Build history of the part. All positions in model axes, mm. A direction names the side the tool comes from. Give positions to 0.01 mm unless a question says otherwise; leave off trailing zeros. Loops run counter-clockwise (first coordinate to the right, second up) from the corner with the lowest first, then second, coordinate; pieces in that order, holes last.
1) Band-saw the part on C-C on y = -3. List the corners of the cut face in (x, z), then the cut area to 3 significant figures.
2) 3-axis set-ups, long thin cutter, end or side, ignore diameter. For faces 1 (the flat face through (0, 0, 15)), 2 (the flat face through (15, 1, -2)), 3 (the flat face through (3.59, 11.248, -11.084)): which of +Z, -Z, +X, -X, +Y, -Y reach the whole face in a straight line?
3) Wall check: line 1 (X direction, y = -3.1, z = 22.45); line 2 (Z direction, x = 0, y = -4.2); line 3 (Z direction, x = 0, y = -3.5). Give the ranges that are in metal, low to high.
4) Band-saw the part on B-B on x = 0. State how many separate pieces and enclosed holes the cut face has, then the cut area to 3 significant figures.
5) Two-plate mould, pull along Y, no slides. Class faces 4 (the flat face through (0.21, 7.314, -6.137)), 5 (the flat face through (0, -2, 30)), 6 (the cylindrical face through (-0.145, 9.063, -8.439)): +Y half, -Y half, draft (parallel to the pull), parting line (faces both ways), or undercut.
6) Band-saw the part on A-A on z = 22.45. List the corners of the cut face in (x, y), then the cut area to 3 significant figures.
7) Flat gauge pins, fed straight in: P1, Ø5, axis at x = -7, z = -0.5, coming from the +Y side; P2, Ø1, axis at y = 3.5, z = -15.5, coming from the -X side; P3, Ø9, axis at x = 4.5, z = 16, coming from the +Y side; P4, Ø2, axis at x = -2, z = -17, coming from the -Y side. Where does each tip first touch, or does it go through?
```python
from build123d import *

# Parameters (mm, degrees)
SKETCH1_W                                           = 30
SKETCH1_H                                           = 5
BOSS_EXTRUDE1_DEPTH                                 = 30
BOSS_EXTRUDE3_DEPTH                                 = 30
CSK_FOR_M4_COUNTERSUNK_FLAT_HEAD_SCREW1_D           = 4.5
CSK_FOR_M4_COUNTERSUNK_FLAT_HEAD_SCREW1_CSINK_D     = 9.4
CSK_FOR_M4_COUNTERSUNK_FLAT_HEAD_SCREW1_CSINK_ANGLE = 90


with BuildPart() as part:
    # Sketch1 → Boss-Extrude1 (new body)
    with BuildSketch(Plane.XY):
        with Locations((0, -2.5)):
            Rectangle(SKETCH1_W, SKETCH1_H)
    extrude(amount=BOSS_EXTRUDE1_DEPTH)

    # Sketch3 → Boss-Extrude3 (add)
    with BuildSketch(Plane(origin=(15, 0, 0), x_dir=(0, 0, -1), z_dir=(1, 0, 0))):
        Polygon((0, 0), (16.069690242, 19.151111078), (26.069690242, 19.151111078), (5.804501844, -5), (0, -5), align=None)
    extrude(amount=-BOSS_EXTRUDE3_DEPTH)

    # Sketch6 → CBORE for M6 Hex Socket Head Cap Screw1 (revolve, cut)
    with BuildSketch(Plane(origin=(0, 7.075555539, -15.937096043), x_dir=(0, 0.766044443, -0.64278761), z_dir=(1, 0, 0))):
        Polygon((0, 0), (0, 42.951874637), (3.3, 42.951874637), (3.3, 6.4), (5.5, 6.4), (5.5, 0.025), (5.525, 0), align=None)
    revolve(axis=Axis((0, 2.993854217, -20.801478257), (0, 0.64278761, 0.766044443)), mode=Mode.SUBTRACT)

    # CSK for M4 Countersunk Flat Head Screw1 (through all)
    with Locations(Plane(origin=(0, 0, 0), x_dir=(1, 0, 0), z_dir=(0, 1, 0))):
        with Locations((0, -7.55), (0, -22.45)):
            CounterSinkHole(CSK_FOR_M4_COUNTERSUNK_FLAT_HEAD_SCREW1_D / 2, CSK_FOR_M4_COUNTERSUNK_FLAT_HEAD_SCREW1_CSINK_D / 2, counter_sink_angle=CSK_FOR_M4_COUNTERSUNK_FLAT_HEAD_SCREW1_CSINK_ANGLE)


solid = part.part
```
Findings below:
1. outline: (-15, -7.48) - (15, -7.48) - (15, 30) - (-15, 30) - close; hole circle Ø4.5 at (0, 7.55); hole circle Ø4.5 at (0, 22.45)
1. area: 1,090 mm2
2. face 1: +Z, +X, -X, +Y
2. face 2: +Z, -Z, +X, +Y, -Y
2. face 3: none
3. line 1: x = -15 to -2.25, 2.25 to 15
3. line 2: z = -6.48 to 5.3, 9.8 to 20.2, 24.7 to 30
3. line 3: z = -7.06 to 5.3, 9.8 to 20.2, 24.7 to 30
4. separate pieces: 4
4. enclosed holes: 0
4. area: 245 mm2
5. face 4: +Y half
5. face 5: draft
5. face 6: undercut
6. outline: (-15, -5) - (-2.25, -5) - (-2.25, -2.45) - (-4.7, 0) - (-15, 0) - close; (2.25, -5) - (15, -5) - (15, 0) - (4.7, 0) - (2.25, -2.45) - close
6. area: 121 mm2
7. P1: stops at y = 3.58
7. P2: passes through
7. P3: stops at y = 0
7. P4: stops at y = 11.84
